Model file for the job. Use its own axes, mm. A direction names the side the tool comes from. Round coordinates to 2 decimals unless told otherwise and drop trailing zeros. Order: outer loops, then holes, each group sorted by start corner. A loop starts at its lowest first (then second) coordinate and runs counter-clockwise, first axis right, second up. Notation, with made-up numbers: (-19.5, 82) - (3.5, 82) arc R22 ccw to (3.5, 120) - close; hole circle Ø1 at (37.5, 68). An arc over 180 degrees is marked (long way). Use one line per item in the form item = value.
from build123d import *

# Parameters (mm, degrees)
F0_W         = 11.5
F0_H         = 6.2
F0_W_2       = 7.5
F0_H_2       = 2.2
F1_DEPTH     = 7
F2_W         = 11.5
F2_H         = 6.2
F3_DEPTH     = 2
F4_R         = 2
F5_R         = 0.8
F6_T1_DEPTH  = 2.2
F6_T3_DEPTH  = 7.5
F6_T6_ANGLE  = 90
F6_T8_ANGLE  = 90
F6_T10_ANGLE = 90
F6_T12_ANGLE = 90


# Not quite as in the source:
# - a fillet or chamfer that OpenCascade refuses, or shapes differently, is made with other operations: its cross-section is extruded or revolved along the edge and cut away or added


with BuildPart() as f1:
    # F0 (on Top) → F1 (new body)
    with BuildSketch(Plane.XY):
        Rectangle(F0_W, F0_H)
        Rectangle(F0_W_2, F0_H_2, mode=Mode.SUBTRACT)
    extrude(amount=F1_DEPTH)

    # F2 (on face) → F3 (join)
    with BuildSketch(Plane(origin=(0, 0, 0), x_dir=(1, 0, 0), z_dir=(0, 0, -1))):
        Rectangle(F2_W, F2_H)
    extrude(amount=F3_DEPTH)

    # F4
    f4_edges = [f1.edges().sort_by_distance(p)[0] for p in [
        (5.75, 0, -2),
        (0, -3.1, -2),
        (-5.75, 0, -2),
        (0, 3.1, -2),
        (5.75, -3.1, 2.5),
        (5.75, 3.1, 2.5),
        (-5.75, -3.1, 2.5),
        (-5.75, 3.1, 2.5),
    ]]
    fillet(f4_edges, radius=F4_R)

    # F5
    f5_edges = [f1.edges().sort_by_distance(p)[0] for p in [
        (0, -1.1, 7),
        (3.75, 0, 7),
        (-3.75, 0, 7),
        (0, 1.1, 7),
    ]]
    fillet(f5_edges, radius=F5_R)

    # F6: fillet of radius 1 on 8 edges, made by hand

    # F6_s2 → F6_t1 (cut)
    with BuildSketch(Plane.XZ.offset(-1.1)):
        with BuildLine():
            ThreePointArc((4.75, 7), (5.4571067812, 6.7071067812), (5.75, 6))
            Line((5.75, 6), (5.75, 7))
            Line((5.75, 7), (4.75, 7))
        make_face()
        with BuildLine():
            ThreePointArc((-4.75, 7), (-5.4571067812, 6.7071067812), (-5.75, 6))
            Line((-5.75, 6), (-5.75, 7))
            Line((-5.75, 7), (-4.75, 7))
        make_face()
    extrude(amount=F6_T1_DEPTH, mode=Mode.SUBTRACT)

    # F6_s4 → F6_t3 (cut)
    with BuildSketch(Plane.YZ.offset(-3.75)):
        with BuildLine():
            ThreePointArc((2.1, 7), (2.8071067812, 6.7071067812), (3.1, 6))
            Line((3.1, 6), (3.1, 7))
            Line((3.1, 7), (2.1, 7))
        make_face()
        with BuildLine():
            ThreePointArc((-2.1, 7), (-2.8071067812, 6.7071067812), (-3.1, 6))
            Line((-3.1, 6), (-3.1, 7))
            Line((-3.1, 7), (-2.1, 7))
        make_face()
    extrude(amount=F6_T3_DEPTH, mode=Mode.SUBTRACT)

    # F6_s5 → F6_t6 (revolve, cut)
    with BuildSketch(Plane.YZ.offset(3.75)):
        with BuildLine():
            ThreePointArc((2.1, 7), (2.8071067812, 6.7071067812), (3.1, 6))
            Line((3.1, 6), (3.1, 7))
            Line((3.1, 7), (2.1, 7))
        make_face()
    revolve(axis=Axis((3.75, 1.1, 7), (0, 0, -1)), revolution_arc=F6_T6_ANGLE, mode=Mode.SUBTRACT)

    # F6_s7 → F6_t8 (revolve, cut)
    with BuildSketch(Plane.YZ.offset(-3.75)):
        with BuildLine():
            ThreePointArc((2.1, 7), (2.8071067812, 6.7071067812), (3.1, 6))
            Line((3.1, 6), (3.1, 7))
            Line((3.1, 7), (2.1, 7))
        make_face()
    revolve(axis=Axis((-3.75, 1.1, 7), (0, 0, 1)), revolution_arc=F6_T8_ANGLE, mode=Mode.SUBTRACT)

    # F6_s9 → F6_t10 (revolve, cut)
    with BuildSketch(Plane.YZ.offset(3.75)):
        with BuildLine():
            ThreePointArc((-2.1, 7), (-2.8071067812, 6.7071067812), (-3.1, 6))
            Line((-3.1, 6), (-3.1, 7))
            Line((-3.1, 7), (-2.1, 7))
        make_face()
    revolve(axis=Axis((3.75, -1.1, 7), (0, 0, 1)), revolution_arc=F6_T10_ANGLE, mode=Mode.SUBTRACT)

    # F6_s11 → F6_t12 (revolve, cut)
    with BuildSketch(Plane.YZ.offset(-3.75)):
        with BuildLine():
            ThreePointArc((-2.1, 7), (-2.8071067812, 6.7071067812), (-3.1, 6))
            Line((-3.1, 6), (-3.1, 7))
            Line((-3.1, 7), (-2.1, 7))
        make_face()
    revolve(axis=Axis((-3.75, -1.1, 7), (0, 0, -1)), revolution_arc=F6_T12_ANGLE, mode=Mode.SUBTRACT)


solid = f1.part
(1) Slice it at A-A on z = 0.75. Give the cut face in (x, y), then the cut area to 3 significant figures.
Report:
outline = (-5.75, -1.1) arc R2 ccw to (-3.75, -3.1) - (3.75, -3.1) arc R2 ccw to (5.75, -1.1) - (5.75, 1.1) arc R2 ccw to (3.75, 3.1) - (-3.75, 3.1) arc R2 ccw to (-5.75, 1.1) - close; hole (-3.75, -1.1) - (3.75, -1.1) - (3.75, 1.1) - (-3.75, 1.1) - close
area = 51.4 mm2
(2) Slice it at B-B on y = -0.5. Give the cut face in (x, z), then the cut area to 3 significant figures.
Report:
outline = (-5.75, 0) arc R2 ccw to (-3.75, -2) - (3.75, -2) arc R2 ccw to (5.75, 0) - (5.75, 6) arc R1 ccw to (4.75, 7) - (4.55, 7) arc R0.8 ccw to (3.75, 6.2) - (3.75, 0) - (-3.75, 0) - (-3.75, 6.2) arc R0.8 ccw to (-4.55, 7) - (-4.75, 7) arc R1 ccw to (-5.75, 6) - close
area = 48.6 mm2
(3) Probe probe 1 along X at (y, z) = (-0.25, 0.75); probe 2 along Y at (x, z) = (-2.5, 5); probe 3 along Z at (x, y) = (3.5, -0.75). List the from-to ranges inside material, lowest first. Write a range as [from, to].
Report:
probe_1 = [-5.75, -3.75], [3.75, 5.75]
probe_2 = [-3.1, -1.1], [1.1, 3.1]
probe_3 = [-2, 0]
(4) Tool access for faces 5 (the face through (-5.75, 0, 3)), 6 (the face through (-3.75, 0, 3)): list every direction of +Z, -Z, +X, -X, +Y, -Y with a clear straight run to the whole face (end or side of a thin tool).
Report:
face_5 = +Z, -Z, -X, +Y, -Y
face_6 = +Z
(5) Pull direction X, two halves, no side cores. Call faces 1 (the face through (5.15, 2.53, 2.96)), 2 (the face through (4.1, 0.03, 6.86)), 3 (the face through (-0.053, -2.799, 6.715)), 4 (the face through (-5.18, -0.02, -1.4)): released by +X, released by -X, zero draft, split by the parting line, or undercut.
Report:
face_1 = released by +X
face_2 = undercut
face_3 = zero draft
face_4 = released by -X
(6) Pin check, flat tips, straight feed: pin 1 (2.5 mm diameter, centred on x = -1.5, y = 0.5, fed in from +Z); pin 2 (2 mm diameter, centred on x = 0.5, y = 0.5, fed in from +Z). Stop position of each tip, or through.
Report:
pin_1 = 6.99
pin_2 = 6.89
(7) Slice it at C-C on x = -0.25. Give the cut face in (y, z), then the cut area to 3 significant figures.
Report:
outline = (-3.1, 0) arc R2 ccw to (-1.1, -2) - (1.1, -2) arc R2 ccw to (3.1, 0) - (3.1, 6) arc R1 ccw to (2.1, 7) - (1.9, 7) arc R0.8 ccw to (1.1, 6.2) - (1.1, 0) - (-1.1, 0) - (-1.1, 6.2) arc R0.8 ccw to (-1.9, 7) - (-2.1, 7) arc R1 ccw to (-3.1, 6) - close
area = 38.0 mm2
